Verification items for the finished model (mm, model axes). A direction names the side the tool comes from. Coordinates: 2 decimals unless noted, no trailing zeros. Order: outer loops, then holes, each group sorted by start corner. A loop starts at its lowest first (then second) coordinate and runs counter-clockwise, first axis right, second up.
Q1. Cross-section at B-B, the plane z = 0. Record the boundary of the cut face in (x, y).
Q2. Draft check along X on faces 4 (the flat face through (19, -4.318, 14)), 5 (the cylindrical face through (1.326, -0.075, -30.133)), 6 (the flat face through (-22, -1.499, 15)). Enter one of: pulls with the +X half, pulls with the -X half, needs draft (parallel to the pull), parting line crosses it, or undercut.
Q3. Depth check by flat-ended pin: P1, Ø4.5, axis at x = 21, z = 13, coming from the +Y side; P2, Ø4, axis at y = 3, z = 5, coming from the +X side; P3, Ø3, axis at y = -2, z = 15, coming from the +X side. Enter the tip coordinate at first touch or a pass-through.
Q4. Cross-section at A-A, the plane x = 0. Record the boundary of the cut face in (y, z).
Q5. Thickness scan on line 1 (X direction, y = 1.75, z = 11); line 2 (Y direction, x = 11, z = 25.5); line 3 (X direction, y = -3, z = 16.5). Record the ranges inside material, lowest first.
Q6. Cross-section at C-C, the plane y = 0. Record the boundary of the cut face in (x, z) (1 decimal), and give its area (3 significant figures).
Q7. Set-up check for faces 1 (the cylindrical face through (-20.329, 1.45, 16.393)), 2 (the cylindrical face through (-16.175, -4.068, 12.685)), 3 (the cylindrical face through (-0.32, -2.928, -21.693)): record each of +Z, -Z, +X, -X, +Y, -Y from which the full face is reachable in a straight line by a thin tool's end or side.
from build123d import *

# Parameters (mm, degrees)
SKETCH1_R                                      = 30.1625
EXTRUDE1_DEPTH                                 = 4.318
CBORE_FOR_8_SOCKET_HEAD_CAP_SCREW1_D           = 4.9149
CBORE_FOR_8_SOCKET_HEAD_CAP_SCREW1_CBORE_D     = 8.73125
CBORE_FOR_8_SOCKET_HEAD_CAP_SCREW1_CBORE_DEPTH = 5.8166
CIRPATTERN1_COUNT                              = 3
SKETCH5_R                                      = 30.1625
SKETCH5_R_2                                    = 4.7625
CUT_EXTRUDE1_DEPTH                             = 0.508
CHAMFER1_SIZE                                  = 0.762


with BuildPart() as part:
    # Sketch1 → Extrude1 (new body, symmetric)
    with BuildSketch(Plane(origin=(0, 0, 0), x_dir=(1, 0, 0), z_dir=(0, 1, 0))):
        with Locations(Location((0, 0, 0), (0, 0, 270))):  # turned: the seam where the file's is
            Circle(SKETCH1_R)
    extrude(amount=EXTRUDE1_DEPTH, both=True)

    # CBORE for _8 Socket Head Cap Screw1 (through all)
    with Locations(Plane(origin=(0, 4.318, 0), x_dir=(-1, 0, 0), z_dir=(0, 1, 0))):
        with Locations((0, -24.13)):
            cbore_for_8_socket_head_cap_screw1 = CounterBoreHole(CBORE_FOR_8_SOCKET_HEAD_CAP_SCREW1_D / 2, CBORE_FOR_8_SOCKET_HEAD_CAP_SCREW1_CBORE_D / 2, CBORE_FOR_8_SOCKET_HEAD_CAP_SCREW1_CBORE_DEPTH)

    # CirPattern1: CBORE for _8 Socket Head Cap Screw1 ×3 about axis
    cirpattern1_axis = Axis((0, 0, 0), (0, 1, 0))
    for i in range(1, CIRPATTERN1_COUNT):
        add(cbore_for_8_socket_head_cap_screw1.rotate(cirpattern1_axis, i * 360 / CIRPATTERN1_COUNT), mode=Mode.SUBTRACT)

    # Sketch5 → Cut-Extrude1 (cut)
    with BuildSketch(Plane.XZ.offset(4.318)):
        with Locations(Location((0, 0, 0), (0, 0, 270))):  # turned: the seam where the file's is
            Circle(SKETCH5_R)
        with Locations(Location((-20.897192993, 12.065, 0), (0, 0, 270))):  # turned: the seam where the file's is
            Circle(SKETCH5_R_2, mode=Mode.SUBTRACT)
        with Locations(Location((0, -24.13, 0), (0, 0, 270))):  # turned: the seam where the file's is
            Circle(SKETCH5_R_2, mode=Mode.SUBTRACT)
        with Locations(Location((20.897192993, 12.065, 0), (0, 0, 270))):  # turned: the seam where the file's is
            Circle(SKETCH5_R_2, mode=Mode.SUBTRACT)
    extrude(amount=-CUT_EXTRUDE1_DEPTH, mode=Mode.SUBTRACT)

    # Chamfer1
    chamfer1_edges = [part.edges().sort_by_distance(p)[0] for p in [
        (0, 4.318, -30.1625),
    ]]
    chamfer(chamfer1_edges, length=CHAMFER1_SIZE)


solid = part.part
Check values:
1. outline: (-30.16, -3.81) - (30.16, -3.81) - (30.16, 3.56) - (29.4, 4.32) - (-29.4, 4.32) - (-30.16, 3.56) - close
2. face 4: needs draft
2. face 5: parting line crosses it
2. face 6: undercut
3. P1: stops at y = -1.5
3. P2: stops at x = 30.01
3. P3: stops at x = 26.97
4. outline: (-4.32, -28.89) - (-3.81, -28.89) - (-3.81, -30.16) - (3.56, -30.16) - (4.32, -29.4) - (4.32, -28.5) - (-1.5, -28.5) - (-1.5, -26.59) - (-4.32, -26.59) - close; (-4.32, -21.67) - (-1.5, -21.67) - (-1.5, -19.76) - (4.32, -19.76) - (4.32, 29.4) - (3.56, 30.16) - (-3.81, 30.16) - (-3.81, -19.37) - (-4.32, -19.37) - close
5. line 1: x = -28.09 to -25.13, -16.66 to 16.66, 25.13 to 28.09
5. line 2: y = -3.81 to 4.32
5. line 3: x = -25.25 to 25.25
6. outline: circle Ø60.3 at (0, 0); hole circle Ø8.7 at (-20.9, 12.1); hole circle Ø8.7 at (0, -24.1); hole circle Ø8.7 at (20.9, 12.1)
6. area: 2,680 mm2
7. face 1: +Y
7. face 2: -Y
7. face 3: +Y, -Y
